from build123d import *

# Parameters (mm, degrees)
CHAMFER_SIZE = 1
FILLET_R     = 10


with BuildPart() as part:
    # Sketch → Revolution (revolve)
    with BuildSketch(Plane.XZ):
        with BuildLine():
            Line((4.136281, 100), (53.643467, 100))
            Line((53.643467, 100), (87.759073, 65.884394))
            Line((87.759073, 65.884394), (87.759073, 52.342683))
            ThreePointArc((87.759073, 52.342683), (89.809326, 47.392936), (94.759073, 45.342683))
            Line((94.759073, 45.342683), (105.666697, 45.342683))
            Line((105.666697, 45.342683), (122.742529, 28.266851))
            Line((122.742529, 28.266851), (122.742529, 10))
            Line((122.742529, 10), (12.136281, 10))
            ThreePointArc((4.136281, 18), (6.479427, 12.343146), (12.136281, 10))
            Line((4.136281, 18), (4.136281, 100))
        make_face()
    revolve(axis=Axis((0, 0, 0), (0, 0, 1)))

    # Chamfer
    chamfer_edges = [part.edges().sort_by_distance(p)[0] for p in [
        (-94.759073, 0, 45.342683),
        (-105.666697, 0, 45.342683),
    ]]
    chamfer(chamfer_edges, length=CHAMFER_SIZE)

    # Fillet
    fillet_edges = [part.edges().sort_by_distance(p)[0] for p in [
        (-4.136281, 0, 100),
        (-53.643467, 0, 100),
    ]]
    fillet(fillet_edges, radius=FILLET_R)


solid = part.part
Could you check a few things on this model? Use its own coordinates, in mm. A direction names the side the tool comes from. Give positions to 0.01 mm unless a question says otherwise; leave off trailing zeros. Order: outer loops, then holes, each group sorted by start corner. A loop starts at its lowest first (then second) coordinate and runs counter-clockwise, first axis right, second up. Notation, with made-up numbers: (-17, 48) -> (8, 48) arc R22 ccw to (8, 63) -> close; hole circle Ø7 at (-0.5, 81.25). An arc over 180 degrees is marked (long way). Answer in a Markdown table with one row per item. Add a question column.
Item 1: Imagine slicing it at D-D (z = 21). List the corners of the cut face in (x, y) for me.
Item 2: We'd pull the mould along X, two halves only. Please class faces 1 (the cylindrical face through (-0.897, -4.038, 54.504)), 2 (the flat face through (16, 94, 45.343)), 3 (the conical face through (-12.69, -57.13, 95.12)): pulls with the +X half, pulls with the -X half, needs draft (parallel to the pull), parting line crosses it, or undercut.
Item 3: Imagine slicing it at A-A (y = 0). List the corners of the cut face in (x, z) for me, and give its area (3 significant figures).
Item 4: Please list where these lines run through material, in increasing order: probe 1 along Z at (x, y) = (88, -42); probe 2 along Y at (x, z) = (0, 70); probe 3 along Y at (x, z) = (0, 68.5).
Item 5: Imagine slicing it at C-C (z = 60). List the corners of the cut face in (x, y) for me.
Item 6: I'm going to push flat-ended pins straight in: P1, Ø12, axis at x = 89.5, y = -91.5, coming from the +Z side; P2, Ø3, axis at x = 75, z = 50, coming from the -Y side; P3, Ø2, axis at y = -28.5, z = 35.5, coming from the +X side; P4, Ø6.5, axis at x = 0, y = 0, coming from the -Z side (3 decimals). Where does each tip first touch, or does it pass through?
Item 7: For faces 4 (the cylindrical face through (-26.608, -119.824, 19.006)), 5 (the cylindrical face through (-19.024, -85.672, 59.019)), which set-ups out of +Z, -Z, +X, -X, +Y, -Y let a thin tool reach every point of the face, with its end or its side?
Result:
| question | item | result |
|---|---|---|
| 1 | outline | circle Ø245.49 at (0, 0); hole circle Ø8.27 at (0, 0) |
| 2 | face 1 | undercut |
| 2 | face 2 | needs draft |
| 2 | face 3 | parting line crosses it |
| 3 | outline | (-122.74, 10) -> (-12.14, 10) arc R8 ccw to (-4.14, 18) -> (-4.14, 90) arc R10 ccw to (-14.14, 100) -> (-49.5, 100) arc R10 ccw to (-56.57, 97.07) -> (-87.76, 65.88) -> (-87.76, 52.34) arc R7 cw to (-94.76, 45.34) -> (-104.67, 45.34) -> (-106.37, 44.64) -> (-122.74, 28.27) -> close; (4.14, 18) arc R8 ccw to (12.14, 10) -> (122.74, 10) -> (122.74, 28.27) -> (106.37, 44.64) -> (104.67, 45.34) -> (94.76, 45.34) arc R7 cw to (87.76, 52.34) -> (87.76, 65.88) -> (56.57, 97.07) arc R10 ccw to (49.5, 100) -> (14.14, 100) arc R10 ccw to (4.14, 90) -> close |
| 3 | area | 16,000 mm2 |
| 4 | probe 1 | 10 to 45.34 |
| 4 | probe 2 | -83.64 to -4.14, 4.14 to 83.64 |
| 4 | probe 3 | -85.14 to -4.14, 4.14 to 85.14 |
| 5 | outline | circle Ø175.52 at (0, 0); hole circle Ø8.27 at (0, 0) |
| 6 | P1 | z = 29.02 |
| 6 | P2 | y = -48.96 |
| 6 | P3 | x = 113 |
| 6 | P4 | through |
| 7 | face 4 | +Z, -Z |
| 7 | face 5 | +Z |
